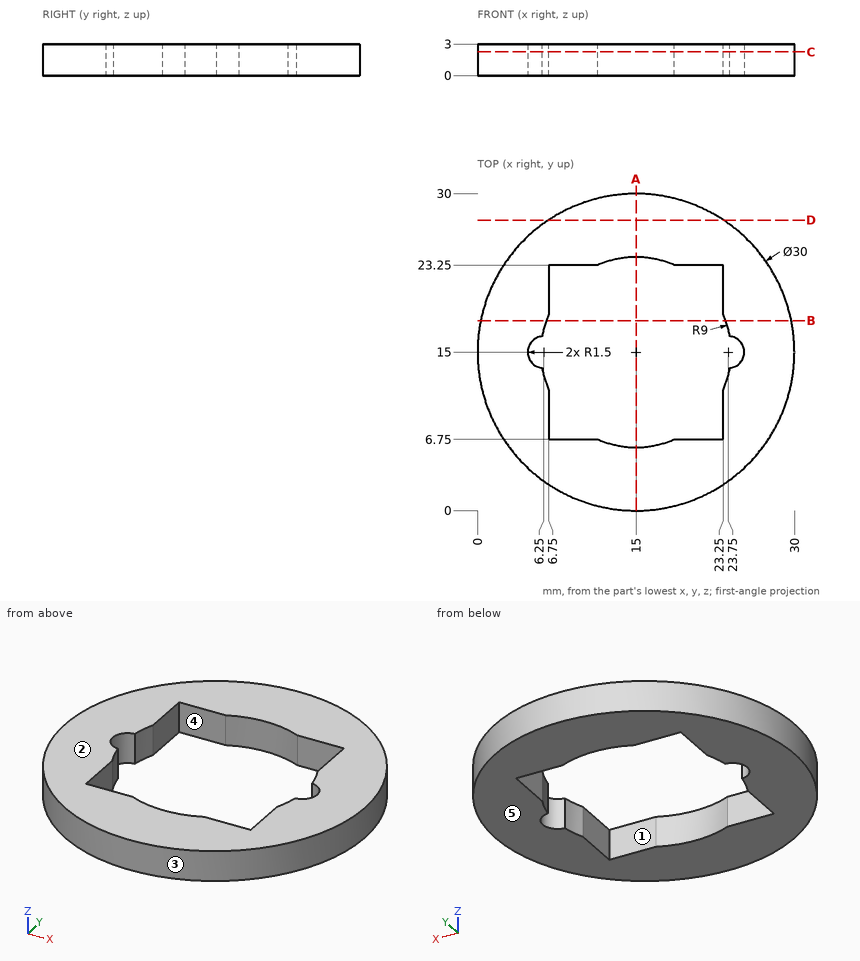
Check sheet for the drawn part. Datum: minimum x, y, z corner. Units: mm. A direction names the side the tool comes from. Give positions to 0.01 mm unless a question says otherwise; leave off trailing zeros. Order: outer loops, then holes, each group sorted by start corner. A loop starts at its lowest first (then second) coordinate and runs counter-clockwise, first axis right, second up. Notation, with made-up numbers: (37.25, 86) -> (52.25, 86) arc R19 cw to (52.25, 98) -> close; hole circle Ø8 at (31, 59.5). An arc over 180 degrees is marked (long way). Answer as CSV lines item,"result".
Q1. Scan lines: probe 1 along X at (y, z) = (9.5, 2.3); probe 2 along Y at (x, z) = (8, 1.6); probe 3 along X at (y, z) = (22.5, 2.35). Record each from-to range of solid material in increasing order.
Solutions:
probe 1,"x = 1.04 to 6.75, 23.25 to 28.96"
probe 2,"y = 1.73 to 6.75, 23.25 to 28.27"
probe 3,"x = 2.01 to 6.75, 23.25 to 27.99"
Q2. Access from +Z, -Z, +X, -X, +Y, -Y to the whole of each face (thin tool, end or side, straight path). Record for the marked faces 4 and 5.
Solutions:
face 4,"+Z, -Z"
face 5,"-Z, +X, -X, +Y, -Y"
Q3. Sectioned sample at A-A on x = 15. Record the cut outline in (y, z).
Solutions:
outline,"(0, 0) -> (6, 0) -> (6, 3) -> (0, 3) -> close; (24, 0) -> (30, 0) -> (30, 3) -> (24, 3) -> close"
Q4. Depth check by flat-ended pin: pin 1 (1.5 mm diameter, centred on y = 8.5, z = 2, fed in from +X); pin 2 (3 mm diameter, centred on x = 12, y = 20, fed in from +Z); pin 3 (1.5 mm diameter, centred on x = 21.5, z = 1, fed in from +Y); pin 4 (1 mm diameter, centred on x = 5, z = 1, fed in from +Y). Enter the tip coordinate at first touch or a pass-through.
Solutions:
pin 1,"stops at x = 28.85"
pin 2,"passes through"
pin 3,"stops at y = 28.85"
pin 4,"stops at y = 26.61"
Q5. Sectioned sample at B-B on y = 18. Record the cut outline in (x, z).
Solutions:
outline,"(0.3, 0) -> (6.51, 0) -> (6.51, 3) -> (0.3, 3) -> close; (23.49, 0) -> (29.7, 0) -> (29.7, 3) -> (23.49, 3) -> close"
Q6. Sectioned sample at D-D on y = 27.5. Record the cut outline in (x, z).
Solutions:
outline,"(6.71, 0) -> (23.29, 0) -> (23.29, 3) -> (6.71, 3) -> close"
Q7. Sectioned sample at C-C on z = 2.25. Record the cut outline in (x, y) (3 decimals).
Solutions:
outline,"circle Ø30 at (15, 15); hole (6.125, 13.505) arc R9 ccw to (6.75, 11.403) -> (6.75, 6.75) -> (11.403, 6.75) arc R9 ccw to (18.597, 6.75) -> (23.25, 6.75) -> (23.25, 11.403) arc R9 ccw to (23.875, 13.505) arc R1.5 ccw to (23.875, 16.495) arc R9 ccw to (23.25, 18.597) -> (23.25, 23.25) -> (18.597, 23.25) arc R9 ccw to (11.403, 23.25) -> (6.75, 23.25) -> (6.75, 18.597) arc R9 ccw to (6.125, 16.495) arc R1.5 ccw to start"
Q8. Release check for a two-part mould opening along Y. For the marked faces 1, 2 and 3 record: +Y half, -Y half, draft (parallel to the pull), parting line (faces both ways), or undercut.
Solutions:
face 1,"undercut"
face 2,"draft"
face 3,"parting line"
